The model under review builds one solid part; all positions refer to its coordinate system, in mm. Face numbers are marked on the shaded views. A direction names the side the tool comes from. Coordinates: 2 decimals unless noted, no trailing zeros. Write each loop counter-clockwise with the first axis right and the second up, starting at its lowest first coordinate (ties: lowest second). Pieces come first, ordered by that corner, then holes.
1) For P1, Ø10, axis at y = 22, z = 22.5, coming from the -X side; P2, Ø6.5, axis at y = 8.5, z = 19.5, coming from the +X side; P3, Ø10, axis at y = 24, z = 10, coming from the -X side, all flat-tipped, find the tip position at first contact; note any pin that passes through.
2) Add section A-A, the plane y = 15. State the section outline as (x, z) points, then the cut area to 3 significant figures.
3) Add section C-C, the plane x = 52. State the section outline as (y, z) points, then the cut area to 3 significant figures.
4) Machinability: for the marked faces 1 and 2, which of the approach directions +Z, -Z, +X, -X, +Y, -Y give a long, thin tool a straight path to every point of the face, cutting with its end or side? Answer none if there is none.
5) Add section B-B, the plane z = 18.5. State the section outline as (x, y) points.
6) Add section D-D, the plane y = 27. State the section outline as (x, z) points, then the cut area to 3 significant figures.
7) For line 1 (Y direction, x = 0, z = 7.75); line 2 (Z direction, x = 32, y = 7.5); line 3 (X direction, y = 18, z = 2.5), list the stretches that pass through material, from the lowest coordinate up.
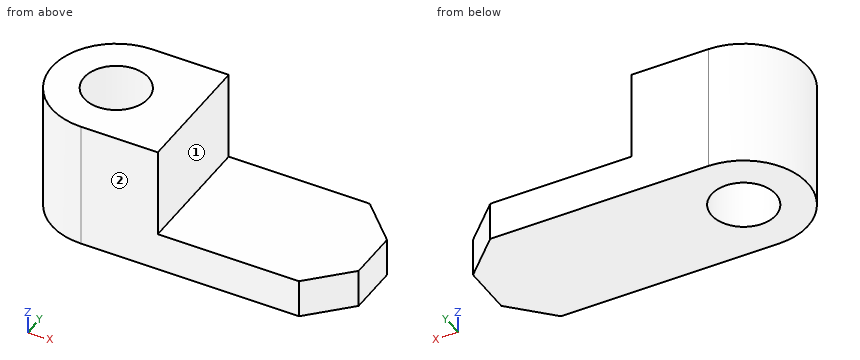
from build123d import *

# Parameters (mm, degrees)
F0_R     = 7.5
F1_DEPTH = 9
F2_R     = 7.5
F3_DEPTH = 21


with BuildPart() as f1:
    # F0 (on Top) → F1 (new body)
    with BuildSketch(Plane.XY):
        with BuildLine():
            ThreePointArc((0, 30), (-15, 15), (0, 0))
            Line((0, 0), (51, 0))
            Line((51, 0), (60, 9))
            Line((60, 9), (60, 21))
            Line((60, 21), (51, 30))
            Line((51, 30), (18, 30))
            Line((18, 30), (0, 30))
        make_face()
        with Locations((0, 15)):
            Circle(F0_R, mode=Mode.SUBTRACT)
    extrude(amount=F1_DEPTH)

    # F2 (on face) → F3 (join)
    with BuildSketch(Plane.XY.offset(9)):
        with BuildLine():
            ThreePointArc((0, 30), (-15, 15), (0, 0))
            Line((0, 0), (18, 0))
            Line((18, 0), (18, 30))
            Line((18, 30), (0, 30))
        make_face()
        with Locations((0, 15)):
            Circle(F2_R, mode=Mode.SUBTRACT)
    extrude(amount=F3_DEPTH)


solid = f1.part
Geometry results:
1. P1: stops at x = -14.87
1. P2: stops at x = 18
1. P3: stops at x = -14.46
2. outline: (-15, 0) - (-7.5, 0) - (-7.5, 30) - (-15, 30) - close; (7.5, 0) - (60, 0) - (60, 9) - (18, 9) - (18, 30) - (7.5, 30) - close
2. area: 918 mm2
3. outline: (1, 0) - (29, 0) - (29, 9) - (1, 9) - close
3. area: 252 mm2
4. face 1: +Z, +X, +Y, -Y
4. face 2: +Z, -Z, +X, -X, -Y
5. outline: (0, 0) - (18, 0) - (18, 30) - (0, 30) arc R15 ccw to start; hole circle Ø15 at (0, 15)
6. outline: (-9, 0) - (54, 0) - (54, 9) - (18, 9) - (18, 30) - (-9, 30) - close
6. area: 1,130 mm2
7. line 1: y = 0 to 7.5, 22.5 to 30
7. line 2: z = 0 to 9
7. line 3: x = -14.7 to -6.87, 6.87 to 60
